Check sheet for the modelled part. Datum: model origin and axes. Units: mm. Round coordinates to 2 decimals unless told otherwise and drop trailing zeros. Write each loop counter-clockwise with the first axis right and the second up, starting at its lowest first coordinate (ties: lowest second). Pieces come first, ordered by that corner, then holes. Notation, with made-up numbers: (-10, -5.5) -> (27, -5.5) arc R7 cw to (27, 4.5) -> close; hole circle Ø7 at (12.5, 71.25). An arc over 180 degrees is marked (long way). One line per item, written item: value.
from build123d import *

# Parameters (mm, degrees)
F0_W     = 121.5
F0_H     = 62
F1_DEPTH = 3
F3_D     = 7.5
F5_D     = 7.5
F7_D     = 7.5


with BuildPart() as f1:
    # F0 (on Top) → F1 (new body)
    with BuildSketch(Plane.XY):
        with Locations((1619.258806, -621.851886)):
            Rectangle(F0_W, F0_H)
    extrude(amount=F1_DEPTH)

    # F3 (through all)
    with Locations(Plane.XY.offset(3)):
        with Locations((1564.258806, -647.101886)):
            Hole(F3_D / 2)

    # F5 (through all)
    with Locations(Plane.XY.offset(3)):
        with Locations((1564.258806, -596.601886)):
            Hole(F5_D / 2)

    # F7 (through all)
    with Locations(Plane.XY.offset(3)):
        with Locations((1674.258806, -596.601886), (1674.258806, -647.101886)):
            Hole(F7_D / 2)


solid = f1.part
Item 1: Sectioned sample at B-B (z = 0.5). Enter the section's corners in (x, y), then the cut area to 3 significant figures.
Result set:
outline: (1558.51, -652.85) -> (1680.01, -652.85) -> (1680.01, -590.85) -> (1558.51, -590.85) -> close; hole circle Ø7.5 at (1564.26, -647.1); hole circle Ø7.5 at (1564.26, -596.6); hole circle Ø7.5 at (1674.26, -647.1); hole circle Ø7.5 at (1674.26, -596.6)
area: 7,360 mm^2
Item 2: Material ranges on line 1 along X through (y, z) = (-649.5, 0.75); line 2 along X through (y, z) = (-600, 2.85), recorded low to high.
Result set:
line 1: 1558.51 to 1561.38, 1567.14 to 1671.38, 1677.14 to 1680.01
line 2: 1558.51 to 1562.67, 1565.84 to 1672.67, 1675.84 to 1680.01
Item 3: Release check for a two-part mould opening along Y. For faces 1 (the cylindrical face through (1567.235, -649.384, 1.479)), 2 (the flat face through (1618, -590.852, 1)), 3 (the flat face through (1618, -621, 0)) record: pulls with the +Y half, pulls with the -Y half, needs draft (parallel to the pull), parting line crosses it, or undercut.
Result set:
face 1: undercut
face 2: pulls with the +Y half
face 3: needs draft
Item 4: Sectioned sample at A-A (y = -645.5). Enter the section's corners in (x, z).
Result set:
outline: (1558.51, 0) -> (1560.87, 0) -> (1560.87, 3) -> (1558.51, 3) -> close; (1567.65, 0) -> (1670.87, 0) -> (1670.87, 3) -> (1567.65, 3) -> close; (1677.65, 0) -> (1680.01, 0) -> (1680.01, 3) -> (1677.65, 3) -> close
